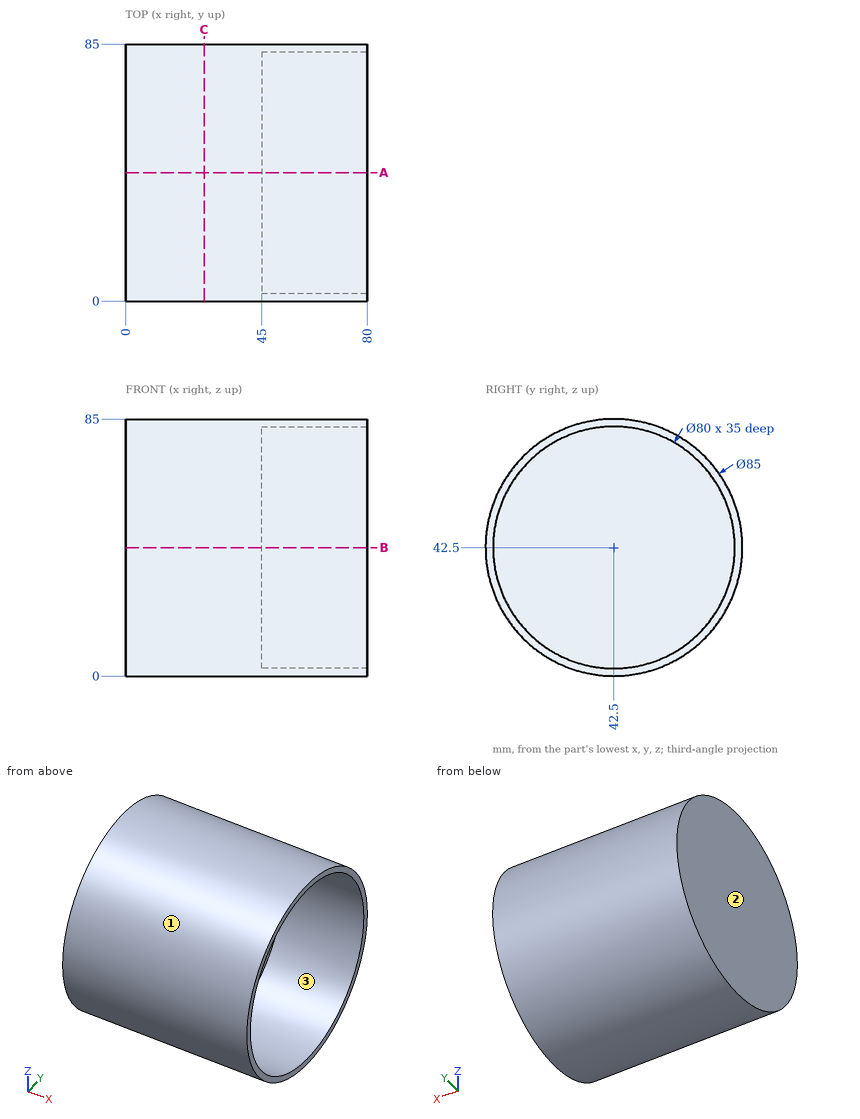
Verification items for this drawing (mm, ordinates from the low corner). Coordinates: 2 decimals unless noted, no trailing zeros. Write each loop counter-clockwise with the first axis right and the second up, starting at its lowest first coordinate (ties: lowest second). Pieces come first, ordered by that corner, then holes. Notation, with made-up numbers: M -21,-38 L 8,-38 A10 ccw 8,-33 Z; hole C 67,38.25 d11. An arc over 180 degrees is marked long. One line per item, written item: value. Start each with the question number.
(1) Sectioned sample at C-C, the plane x = 26. Enter the section's corners in (y, z).
(2) Release check for a two-part mould opening along Y. For the marked faces 1, 2 and 3 record: released by +Y, released by -Y, zero draft, split by the parting line, or undercut.
(3) Sectioned sample at A-A, the plane y = 42.5. Enter the section's corners in (x, z).
(4) Scan lines: line 1 along Z through (x, y) = (70, 42); line 2 along X through (y, z) = (56.5, 19). Record each from-to range of solid material in increasing order. Write a range as [from, to].
(5) Depth check by flat-ended pin: pin 1 (1.5 mm diameter, centred on y = 20.5, z = 32, fed in from +X); pin 2 (2 mm diameter, centred on x = 25, y = 55, fed in from -Z); pin 3 (1 mm diameter, centred on x = 55, z = 57.5, fed in from +Y). Enter the tip coordinate at first touch or a pass-through.
Filled sheet:
1. outline: C 42.5,42.5 d85
2. face 1: split by the parting line
2. face 2: zero draft
2. face 3: undercut
3. outline: M 0,0 L 80,0 L 80,2.5 L 45,2.5 L 45,82.5 L 80,82.5 L 80,85 L 0,85 Z
4. line 1: [0, 2.5], [82.5, 85]
4. line 2: [0, 45]
5. pin 1: x = 45
5. pin 2: z = 1.59
5. pin 3: y = 82.45
